Drawing for the job (mm, zero at the part's lowest x, y, z). A direction names the side the tool comes from. Give positions to 0.01 mm unless a question says otherwise; leave off trailing zeros. Loops run counter-clockwise (first coordinate to the right, second up) from the corner with the lowest first, then second, coordinate; pieces in that order, holes last. Notation, with made-up numbers: (-29.75, 21.25) - (0.25, 21.25) arc R21 cw to (0.25, 41.25) - close; hole circle Ø7 at (40, -24.5). An arc over 180 degrees is marked (long way). Return JSON: item names as keys, results as strings. Group by question number.
1) Drop flat-ended pins along their axis: pin 1 (1.2 mm diameter, centred on x = 10, y = 4.5, fed in from +Z); pin 2 (1.2 mm diameter, centred on x = 1, y = 3, fed in from +Z). Give the stop position or say it passes through.
2) Slice it at A-A (z = 9.75). List the corners of the cut face in (x, y), and give its area (3 significant figures).
3) Drill centre lines: probe 1 along Z at (x, y) = (10.75, 3); probe 2 along X at (y, z) = (5.5, 4.75); probe 3 along Z at (x, y) = (1, 5). Where is each one in solid material? Low to high. Write a range as from..to.
4) 3-axis set-ups, long thin cutter, end or side, ignore diameter. For the marked faces 1 and 2: which of +Z, -Z, +X, -X, +Y, -Y reach the whole face in a straight line?
5) Slice it at B-B (z = 23.25). List the corners of the cut face in (x, y), and give its area (3 significant figures).
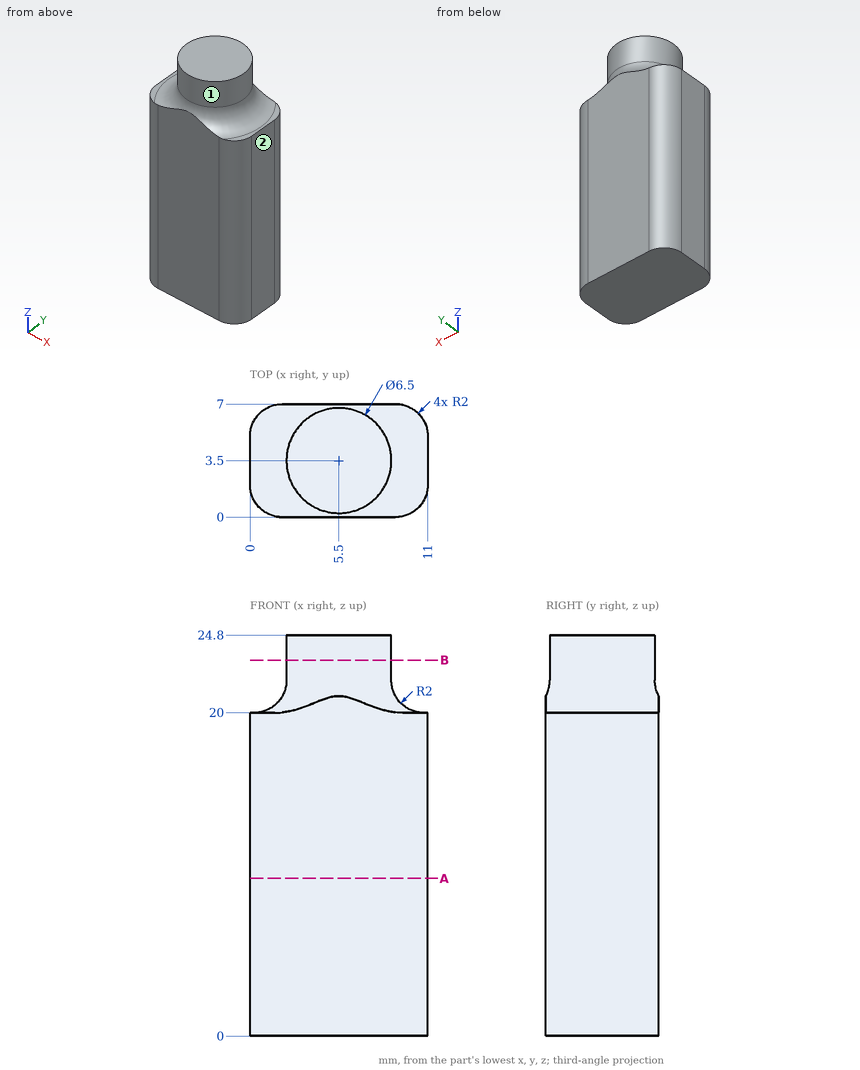
Results:
{
 "1": {"pin 1": "z = 20.43", "pin 2": "z = 20.5"},
 "2": {"outline": "(0, 2) arc R2 ccw to (2, 0) - (9, 0) arc R2 ccw to (11, 2) - (11, 5) arc R2 ccw to (9, 7) - (2, 7) arc R2 ccw to (0, 5) - close", "area": "73.6 mm2"},
 "3": {"probe 1": "0..20", "probe 2": "0.06..10.94", "probe 3": "0..20.07"},
 "4": {"face 1": "+Z", "face 2": "+Z, -Z, +X, +Y, -Y"},
 "5": {"outline": "circle Ø6.5 at (5.5, 3.5)", "area": "33.2 mm2"}
}
